from build123d import *

# Parameters (mm, degrees)
SKETCH1_W           = 42
SKETCH1_H           = 24
BOSS_EXTRUDE1_DEPTH = 3
SKETCH2_W           = 11
SKETCH2_H           = 3
BOSS_EXTRUDE2_DEPTH = 17
SKETCH3_R           = 2.5
CUT_EXTRUDE1_DEPTH  = 52.273774973
SKETCH4_W           = 15
SKETCH4_H           = 18
CUT_EXTRUDE2_DEPTH  = 3
FILLET1_R           = 2
FILLET2_R           = 2
FILLET3_R           = 2
CUT_EXTRUDE3_DEPTH  = 53.345009313


with BuildPart() as part:
    # Sketch1 → Boss-Extrude1 (new body)
    with BuildSketch(Plane(origin=(0, 0, 0), x_dir=(1, 0, 0), z_dir=(0, 1, 0))):
        with Locations((21, 12)):
            Rectangle(SKETCH1_W, SKETCH1_H)
    extrude(amount=BOSS_EXTRUDE1_DEPTH)

    # Sketch2 → Boss-Extrude2 (add)
    with BuildSketch(Plane.XZ):
        with Locations((36.5, -1.5)):
            Rectangle(SKETCH2_W, SKETCH2_H)
        with Locations((36.5, -22.5)):
            Rectangle(SKETCH2_W, SKETCH2_H)
    extrude(amount=BOSS_EXTRUDE2_DEPTH)

    # Sketch3 → Cut-Extrude1 (cut, through all)
    with BuildSketch(Plane.XY):
        with Locations((36.5, -11)):
            Circle(SKETCH3_R)
    extrude(amount=-CUT_EXTRUDE1_DEPTH, mode=Mode.SUBTRACT)

    # Sketch4 → Cut-Extrude2 (cut)
    with BuildSketch(Plane(origin=(0, 3, 0), x_dir=(1, 0, 0), z_dir=(0, 1, 0))):
        with Locations((34.5, 12)):
            Rectangle(SKETCH4_W, SKETCH4_H)
    extrude(amount=-CUT_EXTRUDE2_DEPTH, mode=Mode.SUBTRACT)

    # Fillet1
    fillet1_edges = [part.edges().sort_by_distance(p)[0] for p in [
        (0, 1.5, -24),
        (0, 1.5, 0),
    ]]
    fillet(fillet1_edges, radius=FILLET1_R)

    # Fillet2
    fillet2_edges = [part.edges().sort_by_distance(p)[0] for p in [
        (42, 3, -1.5),
        (42, -17, -1.5),
        (31, -17, -1.5),
        (42, -17, -22.5),
        (31, -17, -22.5),
        (42, 3, -22.5),
    ]]
    fillet(fillet2_edges, radius=FILLET2_R)

    # Fillet3
    fillet3_edges = [part.edges().sort_by_distance(p)[0] for p in [
        (31, 0, -1.5),
        (31, 0, -22.5),
    ]]
    fillet(fillet3_edges, radius=FILLET3_R)

    # Sketch6 → Cut-Extrude3 (cut, through all)
    with BuildSketch(Plane(origin=(0, 3, 0), x_dir=(1, 0, 0), z_dir=(0, 1, 0))):
        with BuildLine():
            Line((3.3, 20.8), (23.7, 20.8))
            ThreePointArc((23.7, 20.8), (25, 19.5), (23.7, 18.2))
            Line((23.7, 18.2), (3.3, 18.2))
            ThreePointArc((3.3, 18.2), (2, 19.5), (3.3, 20.8))
        make_face()
        with BuildLine():
            Line((3.3, 5.8), (23.7, 5.8))
            ThreePointArc((23.7, 5.8), (25, 4.5), (23.7, 3.2))
            Line((23.7, 3.2), (3.3, 3.2))
            ThreePointArc((3.3, 3.2), (2, 4.5), (3.3, 5.8))
        make_face()
    extrude(amount=-CUT_EXTRUDE3_DEPTH, mode=Mode.SUBTRACT)


solid = part.part
For this review, take the finished solid that the model builds, in its own axes (mm). A direction names the side the tool comes from. Round coordinates to 2 decimals unless told otherwise and drop trailing zeros. Loops run counter-clockwise (first coordinate to the right, second up) from the corner with the lowest first, then second, coordinate; pieces in that order, holes last. Notation, with made-up numbers: (-17, 43) - (-7, 43) arc R19 cw to (-7, 76) - close; hole circle Ø2 at (67, 58.25). An arc over 180 degrees is marked (long way). One line per question, with ' | ' between items.
Q1. Take a section at B-B (z = -19.5). Give the boundary of the cut face in (x, y), and give its area (3 significant figures).
Taken from the geometry:
outline: (0, 0) - (2, 0) - (2, 3) - (0, 3) - close; (25, 0) - (27, 0) - (27, 3) - (25, 3) - close | area: 12.0 mm²
Q2. Tool access review of faces 1 (the flat face through (14, 0, -12)), 2 (the cylindrical face through (38.81, -11.96, -22.48)), 3 (the cylindrical face through (2, 1.5, -19.5)): name each direction out of +Z, -Z, +X, -X, +Y, -Y from which nothing blocks a thin tool from reaching the whole face with its end or side.
Taken from the geometry:
face 1: +Z, -Z, -X, -Y | face 2: +Z, -Z | face 3: +Y, -Y
Q3. For pin 1 (3 mm diameter, centred on y = -6, z = -4, fed in from -X); pin 2 (0.9 mm diameter, centred on y = 1, z = -7.5, fed in from +X), all flat-tipped, find the tip position at first contact; note any pin that passes through.
Taken from the geometry:
pin 1: stops at x = 31 | pin 2: stops at x = 27
Q4. The part is to be moulded in two halves that separate along Z. For faces 4 (the cylindrical face through (31.57, -16.4, -22.48)), 5 (the flat face through (14, 2, -3.2)), 6 (the flat face through (32, -4, 0)), say which applies: released by +Z, released by -Z, zero draft, split by the parting line, or undercut.
Taken from the geometry:
face 4: zero draft | face 5: undercut | face 6: released by +Z
Q5. For line 1 along Z through (x, y) = (17, 0.5); line 2 along Y through (x, z) = (36.5, -0.6); line 3 along Z through (x, y) = (37, -13.75), list the stretches that pass through material, from the lowest coordinate up. Write a range as [from, to].
Taken from the geometry:
line 1: z = [-24, -20.8], [-18.2, -5.8], [-3.2, 0] | line 2: y = [-17, -13.5], [-8.5, 3] | line 3: z = [-24, -21], [-3, 0]
Q6. Take a section at A-A (y = -3.5). Give the boundary of the cut face in (x, z), and give its area (3 significant figures).
Taken from the geometry:
outline: (31, -24) - (42, -24) - (42, -21) - (31, -21) - close; (31, -3) - (42, -3) - (42, 0) - (31, 0) - close | area: 66.0 mm²
Q7. Take a section at D-D (x = 17). Give the boundary of the cut face in (y, z), and give its area (3 significant figures).
Taken from the geometry:
outline: (0, -24) - (3, -24) - (3, -20.8) - (0, -20.8) - close; (0, -18.2) - (3, -18.2) - (3, -5.8) - (0, -5.8) - close; (0, -3.2) - (3, -3.2) - (3, 0) - (0, 0) - close | area: 56.4 mm²
Q8. Take a section at C-C (y = -9). Give the boundary of the cut face in (x, z), and give its area (3 significant figures).
Taken from the geometry:
outline: (31, -24) - (35, -24) - (35, -21) - (31, -21) - close; (31, -3) - (35, -3) - (35, 0) - (31, 0) - close; (38, -24) - (42, -24) - (42, -21) - (38, -21) - close; (38, -3) - (42, -3) - (42, 0) - (38, 0) - close | area: 48.0 mm²
